```python
from build123d import *

# Parameters (mm, degrees)
SZKIC1_R                    = 4
DODANIE_WYCI_GNI_CIE1_DEPTH = 4


with BuildPart() as part:
    # Szkic1 → Dodanie-wyciągnięcie1 (new body)
    with BuildSketch(Plane.XY):
        Polygon((6.5, 3.75277675), (0, 7.505553499), (-6.5, 3.75277675), (-6.5, -3.75277675), (0, -7.505553499), (6.5, -3.75277675), align=None)
        Circle(SZKIC1_R, mode=Mode.SUBTRACT)
    extrude(amount=DODANIE_WYCI_GNI_CIE1_DEPTH)

    # Szkic2 → Wycięcie-obrót1 (revolve, cut)
    with BuildSketch(Plane(origin=(0, 0, 0), x_dir=(1, 0, 0), z_dir=(0, 1, 0))):
        Polygon((-9.964101615, -4), (-6.5, -4), (-9.964101615, -2), align=None)
        Polygon((-9.964101615, -2), (-6.5, 0), (-9.964101615, 0), align=None)
    revolve(axis=Axis((0, 0, 9.891098034), (0, 0, -1)), mode=Mode.SUBTRACT)


solid = part.part
```
Design review of the part built by this model. Coordinates are the model's own, in mm. Round coordinates to 2 decimals unless told otherwise and drop trailing zeros. Write each loop counter-clockwise with the first axis right and the second up, starting at its lowest first coordinate (ties: lowest second). Pieces come first, ordered by that corner, then holes.
Item 1: The part is to be moulded in two halves that separate along Y. For faces 1 (the conical face through (-0.02, 6.74, 3.86)), 2 (the flat face through (3, 3, 4)), 3 (the cylindrical face through (-0.867, -3.905, 1.972)), 4 (the conical face through (5.85, -3.36, 3.86)), say which applies: +Y half, -Y half, draft (parallel to the pull), parting line (faces both ways), or undercut.
Item 2: Clearance check with flat-ended pins moving along their axes: pin 1 Ø1.5 at (x, z) = (-5, 2) entering from +Y; pin 2 Ø2 at (x, z) = (3, 1.5) entering from -Y. State where each tip first meets the part, or that it passes through.
Item 3: For probe 1 along X at (y, z) = (0.25, 1.85); probe 2 along Y at (x, z) = (3, 1.65); probe 3 along Y at (x, z) = (1, 2.95), list the stretches that pass through material, from the lowest coordinate up.
Item 4: We need section A-A on z = 0.9. Write out the cut boundary in (x, y).
Returned:
1. face 1: +Y half
1. face 2: draft
1. face 3: undercut
1. face 4: -Y half
2. pin 1: stops at y = 5.05
2. pin 2: stops at y = -6.35
3. probe 1: x = -6.5 to -3.99, 3.99 to 6.5
3. probe 2: y = -5.77 to -2.65, 2.65 to 5.77
3. probe 3: y = -6.93 to -3.87, 3.87 to 6.93
4. outline: (-6.5, -3.75) - (0, -7.51) - (6.5, -3.75) - (6.5, 3.75) - (0, 7.51) - (-6.5, 3.75) - close; hole circle Ø8 at (0, 0)
